Check sheet for the modelled part. Datum: model origin and axes. Units: mm. A direction names the side the tool comes from. Give positions to 0.01 mm unless a question says otherwise; leave off trailing zeros. Loops run counter-clockwise (first coordinate to the right, second up) from the corner with the lowest first, then second, coordinate; pieces in that order, holes last. Notation, with made-up numbers: (-36.75, 47.25) - (-2.75, 47.25) arc R28 ccw to (-2.75, 75.25) - close; hole circle Ø6 at (-16, 17.25). An arc over 180 degrees is marked (long way). Use CSV: the item, a comma, the result in double quotes.
from build123d import *

# Parameters (mm, degrees)
EXTRUDE_1_DEPTH     = 5.1
CUT_EXTRUDE_1_DEPTH = 10
SWEEP_START         = -0.969556918
SWEEP_2_OUTLINE_W   = 12
SWEEP_2_OUTLINE_H   = 9
SWEEP_2_DEPTH       = 0.969556918
SWEEP_START_2       = -16.13744627
SWEEP_3_OUTLINE_W   = 12
SWEEP_3_OUTLINE_H   = 9
SWEEP_3_DEPTH       = 0.969556918
FILLET_2_R          = 0.4
SKETCH_13_R         = 2.9
CUT_EXTRUDE_3_DEPTH = 2.5
SKETCH_14_R         = 2.1
CUT_EXTRUDE_4_DEPTH = 20.917083723


# Read off the part's stored shape, not the designer's step: 切除-扫描2, 切除-扫描3
with BuildPart() as part:
    # 草图1 → 凸台-拉伸1 (new body)
    with BuildSketch(Plane.XY):
        Polygon((0, 0), (9.525, -0.83332952), (9.525, -17.33332952), (0, -16.5), align=None)
    extrude(amount=EXTRUDE_1_DEPTH)

    # 草图4 → 切除-拉伸1 (cut, symmetric)
    with BuildSketch(Plane(origin=(0, -8.25, 0), x_dir=(1, 0, 0), z_dir=(0, 1, 0))):
        Polygon((0, -5.1), (0.991339577, 0), (0, 0), align=None)
        Polygon((9.525, -5.1), (8.533660423, 0), (9.525, 0), align=None)
    extrude(amount=CUT_EXTRUDE_1_DEPTH, both=True, mode=Mode.SUBTRACT)

    # 切除-扫描2 outline → 切除-扫描2 (cut)
    with BuildSketch(Plane(origin=(0, 0, 0), x_dir=(0.9963324805819772, -0.08399418565625866, 0.016326815773634484), z_dir=(0.08556627920719848, 0.9780270466911105, -0.19010919968086795)).offset(SWEEP_START)):
        with Locations((5, -2.5)):
            Rectangle(SWEEP_2_OUTLINE_W, SWEEP_2_OUTLINE_H)
    extrude(amount=SWEEP_2_DEPTH, mode=Mode.SUBTRACT)

    # 切除-扫描3 outline → 切除-扫描3 (cut)
    with BuildSketch(Plane(origin=(0, 0, 0), x_dir=(0.9963324805819772, -0.08399418565625832, -0.016326815773633797), z_dir=(0.08556627920719802, 0.978027046691112, 0.190109199680861)).offset(SWEEP_START_2)):
        with Locations((6, -5.5)):
            Rectangle(SWEEP_3_OUTLINE_W, SWEEP_3_OUTLINE_H)
    extrude(amount=SWEEP_3_DEPTH, mode=Mode.SUBTRACT)

    # 圆角2
    fillet_2_edges = [part.edges().sort_by_distance(p)[0] for p in [
        (9.029330212, -16.794294244, 2.55),
    ]]
    fillet(fillet_2_edges, radius=FILLET_2_R)

    # 草图13 → 切除-拉伸3 (cut)
    with BuildSketch(Plane.XY.offset(5.1)):
        with Locations((4.7625, -8.25)):
            Circle(SKETCH_13_R)
    extrude(amount=-CUT_EXTRUDE_3_DEPTH, mode=Mode.SUBTRACT)

    # 草图14 → 切除-拉伸4 (cut, through all)
    with BuildSketch(Plane.XY.offset(2.6)):
        with Locations((4.7625, -8.25)):
            Circle(SKETCH_14_R)
    extrude(amount=-CUT_EXTRUDE_4_DEPTH, mode=Mode.SUBTRACT)


solid = part.part
1. Sectioned sample at B-B, the plane x = 4.5. Record the boundary of the cut face in (y, z), and give its area (3 significant figures).
Completed:
outline,"(-16.89, 5.1) - (-15.9, 0) - (-10.33, 0) - (-10.33, 2.6) - (-11.14, 2.6) - (-11.14, 5.1) - close; (-6.17, 0) - (-1.39, 0) - (-0.39, 5.1) - (-5.36, 5.1) - (-5.36, 2.6) - (-6.17, 2.6) - close"
area,"53.8 mm²"
2. Sectioned sample at C-C, the plane x = 7.25. Record the boundary of the cut face in (y, z), and give its area (3 significant figures).
Completed:
outline,"(-17.13, 5.1) - (-16.14, 0) - (-1.63, 0) - (-0.63, 5.1) - (-6.76, 5.1) - (-6.76, 2.6) - (-9.74, 2.6) - (-9.74, 5.1) - close"
area,"71.6 mm²"
3. Sectioned sample at D-D, the plane y = -11.75. Record the boundary of the cut face in (x, z) (3 decimals).
Completed:
outline,"(0, 5.1) - (0.991, 0) - (8.534, 0) - (9.525, 5.1) - close"
4. Set-up check for faces 1 (the face through (6.95, -10.45, 5.1)), 2 (the face through (6.322, -5.805, 3.867)): record each of +Z, -Z, +X, -X, +Y, -Y from which the full face is reachable in a straight line by a thin tool's end or side.
Completed:
face 1,"+Z, +X, -X, +Y, -Y"
face 2,"+Z"
5. Go/stop test with flat-tipped pins: pin 1 Ø1 at (y, z) = (-11.5, 4.5) entering from +X; pin 2 Ø3.5 at (x, y) = (4.76, -8.25) entering from +Z; pin 3 Ø2 at (y, z) = (-14.5, 0.5) entering from +X; pin 4 Ø5 at (x, y) = (4.76, -8.25) entering from +Z. Record where each tip stops, or that it passes through.
Completed:
pin 1,"stops at x = 9.51"
pin 2,"passes through"
pin 3,"stops at x = 8.83"
pin 4,"stops at z = 2.6"
6. Scan lines: line 1 along X through (y, z) = (-9.25, 1.9); line 2 along Y through (x, z) = (6.25, 1.6); line 3 along Z through (x, y) = (7.5, -7.5). Record each from-to range of solid material in increasing order.
Completed:
line 1,"x = 0.62 to 2.92, 6.61 to 8.9"
line 2,"y = -16.37 to -9.73, -6.77 to -1.23"
line 3,"z = 0 to 2.6"
7. Sectioned sample at A-A, the plane y = -8.25. Record the boundary of the cut face in (x, z) (1 decimal).
Completed:
outline,"(0, 5.1) - (1, 0) - (2.7, 0) - (2.7, 2.6) - (1.9, 2.6) - (1.9, 5.1) - close; (6.9, 0) - (8.5, 0) - (9.5, 5.1) - (7.7, 5.1) - (7.7, 2.6) - (6.9, 2.6) - close"
8. Release check for a two-part mould opening along X. For faces 3 (the face through (4.696, -0.912, 2.52)), 4 (the face through (7, -7, 2.6)), 5 (the face through (4.489, -6.168, 1.318)), 6 (the face through (3, -10, 0)) record: released by +X, released by -X, zero draft, split by the parting line, or undercut.
Completed:
face 3,"released by +X"
face 4,"undercut"
face 5,"undercut"
face 6,"zero draft"
